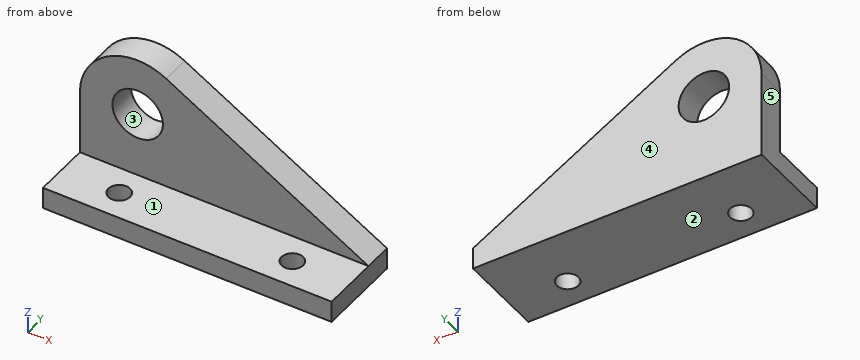
```python
from build123d import *

# Parameters (mm, degrees)
F0_W     = 127
F0_H     = 9.525
F1_DEPTH = 19.05
F3_DEPTH = 12.7
F5_D     = 22.225
F7_D     = 9.525


with BuildPart() as f1:
    # F0 (on Front) → F1 (new body, symmetric)
    with BuildSketch(Plane.XZ):
        Rectangle(F0_W, F0_H)
    extrude(amount=F1_DEPTH, both=True)

    # F2 (on face) → F3 (join)
    with BuildSketch(Plane(origin=(0, 19.05, 0), x_dir=(-1, 0, 0), z_dir=(0, 1, 0))):
        with BuildLine():
            Line((38.1, 4.7625), (63.5, 4.7625))
            Line((63.5, 4.7625), (63.5, 33.3375))
            ThreePointArc((63.5, 33.3375), (50.870136, 55.293903), (25.540659, 55.415157))
            Line((25.540659, 55.415157), (-63.5, 4.7625))
            Line((-63.5, 4.7625), (38.1, 4.7625))
        make_face()
    extrude(amount=-F3_DEPTH)

    # F5 (through all)
    with Locations(Plane.XZ.offset(-6.35)):
        with Locations((-38.1, 33.3375)):
            Hole(F5_D / 2)

    # F7 (through all)
    with Locations(Plane.XY.offset(4.7625)):
        with Locations((-38.1, -6.35), (38.1, -6.35)):
            Hole(F7_D / 2)


solid = f1.part
```
The model under review builds one solid part; all positions refer to its coordinate system, in mm. Face numbers are marked on the shaded views. A direction names the side the tool comes from. Give positions to 0.01 mm unless a question says otherwise; leave off trailing zeros. Write each loop counter-clockwise with the first axis right and the second up, starting at its lowest first coordinate (ties: lowest second). Pieces come first, ordered by that corner, then holes. Notation, with made-up numbers: M -26.75,73 L 6.25,73 A18 cw 6.25,93 Z; hole C 34,87.25 d4. An arc over 180 degrees is marked long. Answer in a Markdown table with one row per item.
Item 1: For P1, Ø1, axis at x = -13.5, y = 2.5, coming from the +Z side; P2, Ø5.5, axis at x = -38.1, y = -6.35, coming from the -Z side; P3, Ø4, axis at x = 25.5, z = 14, coming from the -Y side, all flat-tipped, find the tip position at first contact; note any pin that passes through.
Check sheet entries:
| item | result |
|---|---|
| P1 | z = 4.76 |
| P2 | through |
| P3 | y = 6.35 |
Item 2: For line 1 along X through (y, z) = (-6, 1); line 2 along Y through (x, z) = (-38.1, -0.5), list the stretches that pass through material, from the lowest coordinate up.
Check sheet entries:
| item | result |
|---|---|
| line 1 | -63.5 to -42.85, -33.35 to 33.35, 42.85 to 63.5 |
| line 2 | -19.05 to -11.11, -1.59 to 19.05 |
Item 3: Add section C-C on x = -38.1. State how many separate pieces and enclosed holes the cut face has, plus the area to 3 significant figures.
Check sheet entries:
| item | result |
|---|---|
| separate pieces | 3 |
| enclosed holes | 0 |
| area | 675 mm2 |
Item 4: Add section A-A on y = -6.35. Give the boundary of the cut face in (x, z).
Check sheet entries:
| item | result |
|---|---|
| outline | M -63.5,-4.76 L -42.86,-4.76 L -42.86,4.76 L -63.5,4.76 Z; M -33.34,-4.76 L 33.34,-4.76 L 33.34,4.76 L -33.34,4.76 Z; M 42.86,-4.76 L 63.5,-4.76 L 63.5,4.76 L 42.86,4.76 Z |
Item 5: Add section B-B on z = 37.5. Give the boundary of the cut face in (x, y).
Check sheet entries:
| item | result |
|---|---|
| outline | M -63.16,6.35 L -48.4,6.35 L -48.4,19.05 L -63.16,19.05 Z; M -27.8,6.35 L 5.95,6.35 L 5.95,19.05 L -27.8,19.05 Z |
Item 6: Draft analysis for pull direction X (two halves, no side actions). For the marked faces 3, 4 and 5, state which applies: +X half, -X half, draft (parallel to the pull), parting line (faces both ways), or undercut.
Check sheet entries:
| item | result |
|---|---|
| face 3 | undercut |
| face 4 | draft |
| face 5 | -X half |
Item 7: Tool access review of the marked faces 1 and 2: name each direction out of +Z, -Z, +X, -X, +Y, -Y from which nothing blocks a thin tool from reaching the whole face with its end or side.
Check sheet entries:
| item | result |
|---|---|
| face 1 | +Z, +X, -X, -Y |
| face 2 | -Z, +X, -X, +Y, -Y |
Item 8: Add section D-D on x = 39. Give the boundary of the cut face in (y, z), plus the area to 3 significant figures.
Check sheet entries:
| item | result |
|---|---|
| outline | M -19.05,-4.76 L -11.03,-4.76 L -11.03,4.76 L -19.05,4.76 Z; M -1.67,-4.76 L 19.05,-4.76 L 19.05,18.7 L 6.35,18.7 L 6.35,4.76 L -1.67,4.76 Z |
| area | 451 mm2 |
